The listing builds one solid part. Answer for the finished solid, in the listing's coordinates (mm). A direction names the side the tool comes from. Give positions to 0.01 mm unless a question says otherwise; leave off trailing zeros. Loops run counter-clockwise (first coordinate to the right, second up) from the corner with the lowest first, then second, coordinate; pieces in that order, holes last.
Item 1: Section C-C, the plane y = 37.5 is taken. Give the vertices of the cut face in (x, z), and give its area (3 significant figures).
Item 2: Each of these flat-tipped pins is pushed along its axis until it touches: pin 1 Ø1 at (y, z) = (39, 6.5) entering from -X; pin 2 Ø1 at (x, z) = (-1, 30) entering from -Y; pin 3 Ø2 at (x, y) = (-1.5, 18) entering from +Z. Where does it stop, or does it pass through?
Item 3: Section B-B, the plane y = 18.5 is taken. Give the vertices of the cut face in (x, z), and give its area (3 significant figures).
Item 4: Section A-A, the plane z = 27.52 is taken. Give the vertices of the cut face in (x, y) (3 decimals).
Item 5: Consider line 1 along X through (y, z) = (50.5, 37.5). Determine where the line is inside the solid, lowest interval first.
Item 6: A tool of negligible diameter and unlimited length cuts with its end or side. For faces 5 (the face through (-1, 15, 39.3)), 6 (the face through (-1.01, 26.34, 37.8)), 7 (the face through (-1, 26.3, 17.2)), 8 (the face through (-1, 27.77, 27)), 9 (the face through (-1.01, 3.43, 17.24)), from which of +Z, -Z, +X, -X, +Y, -Y can it reach the whole face along a straight path? Write none if from no direction.
Item 7: Section D-D, the plane z = 13 is taken. Give the vertices of the cut face in (x, y).
Item 8: The mould has two halves that part along Z. Classify faces 1 (the face through (-1, 15, 15.74)), 2 (the face through (11, 60, 20)), 3 (the face through (-0.986, 16.057, 36.443)), 4 (the face through (-1.01, 3.5, 37.87)): pulls with the +Z half, pulls with the -Z half, needs draft (parallel to the pull), parting line crosses it, or undercut.
from build123d import *

# Parameters (mm, degrees)
F0_W     = 60
F0_H     = 41.3
F1_DEPTH = 22.6
F2_R     = 1
F3_W     = 25.77
F3_H     = 23.56
F3_R     = 9
F4_DEPTH = 2
F5_R     = 5


with BuildPart() as f1:
    # F0 (on Right) → F1 (new body)
    with BuildSketch(Plane.YZ):
        with Locations((30, 20.65)):
            Rectangle(F0_W, F0_H)
    extrude(amount=F1_DEPTH)

    # F2
    f2_edges = [f1.edges().sort_by_distance(p)[0] for p in [
        (11.3, 60, 41.3),
        (11.3, 0, 41.3),
        (11.3, 0, 0),
        (11.3, 60, 0),
    ]]
    fillet(f2_edges, radius=F2_R)

    # F3 (on face) → F4 (join)
    with BuildSketch(Plane(origin=(0, 0, 0), x_dir=(0, -1, 0), z_dir=(-1, 0, 0))):
        with Locations((-14.885, 27.52)):
            Rectangle(F3_W, F3_H)
        with Locations((-14.885, 27.52)):
            Circle(F3_R, mode=Mode.SUBTRACT)
    extrude(amount=F4_DEPTH)

    # F5
    f5_edges = [f1.edges().sort_by_distance(p)[0] for p in [
        (-1, 2, 39.3),
        (-1, 2, 15.74),
        (-1, 27.77, 15.74),
        (-1, 27.77, 39.3),
    ]]
    fillet(f5_edges, radius=F5_R)


solid = f1.part
Worked answers:
1. outline: (0, 0) - (22.6, 0) - (22.6, 41.3) - (0, 41.3) - close
1. area: 933 mm2
2. pin 1: stops at x = 0
2. pin 2: stops at y = 2
2. pin 3: stops at z = 39.3
3. outline: (-2, 15.74) - (0, 15.74) - (0, 0) - (22.6, 0) - (22.6, 41.3) - (0, 41.3) - (0, 39.3) - (-2, 39.3) - (-2, 35.76) - (0, 35.76) - (0, 19.28) - (-2, 19.28) - close
3. area: 948 mm2
4. outline: (-2, 2) - (0, 2) - (0, 0) - (22.6, 0) - (22.6, 60) - (0, 60) - (0, 27.77) - (-2, 27.77) - (-2, 23.885) - (0, 23.885) - (0, 5.885) - (-2, 5.885) - close
5. line 1: x = 0 to 22.6
6. face 5: +Z, -X, +Y, -Y
6. face 6: +Z, -X, +Y
6. face 7: -Z, -X, +Y
6. face 8: +Z, -Z, -X, +Y
6. face 9: -Z, -X, -Y
7. outline: (0, 0) - (22.6, 0) - (22.6, 60) - (0, 60) - close
8. face 1: pulls with the -Z half
8. face 2: needs draft
8. face 3: undercut
8. face 4: pulls with the +Z half
